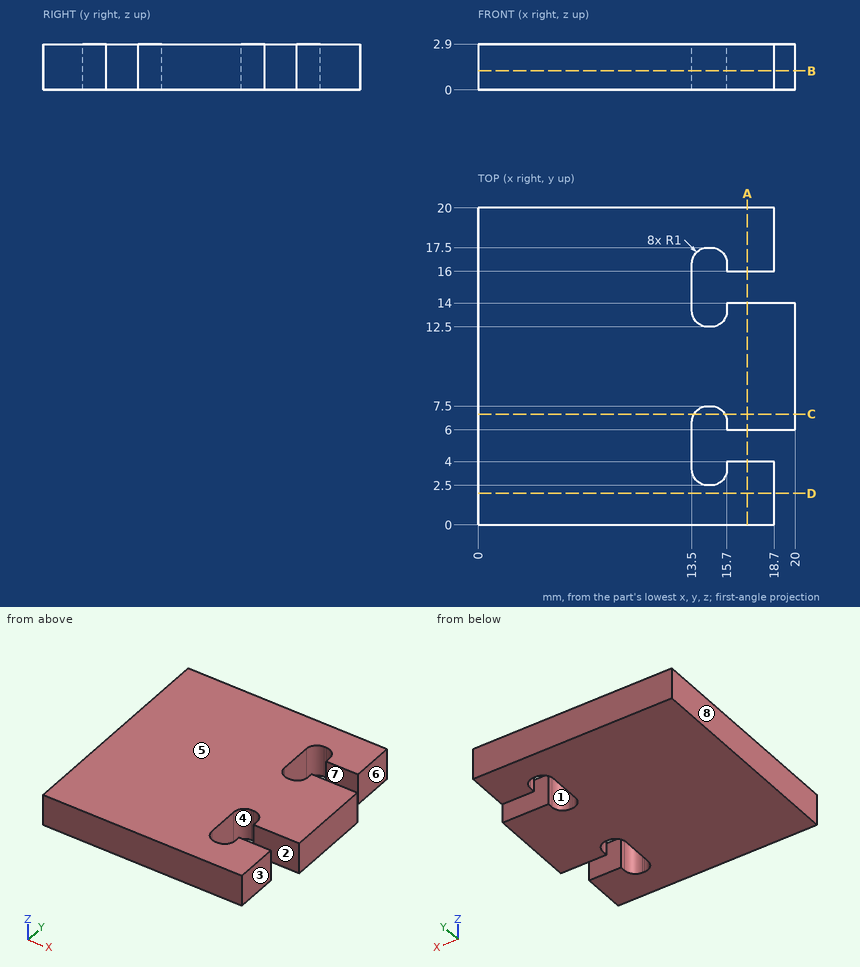
Source: three-view drawing plus pictorial views. Frame: mm from the lowest corner of the part. A direction names the side the tool comes from. Coordinates: 2 decimals unless noted, no trailing zeros. Order: outer loops, then holes, each group sorted by start corner. A loop starts at its lowest first (then second) coordinate and runs counter-clockwise, first axis right, second up.
Item 1: Cut plane B-B (z = 1.2). Return loops of the section in (x, y).
Output values:
outline: (0, 0) - (18.7, 0) - (18.7, 4) - (15.7, 4) - (15.7, 3.5) arc R1 cw to (14.7, 2.5) - (14.5, 2.5) arc R1 cw to (13.5, 3.5) - (13.5, 6.5) arc R1 cw to (14.5, 7.5) - (14.7, 7.5) arc R1 cw to (15.7, 6.5) - (15.7, 6) - (20, 6) - (20, 14) - (15.7, 14) - (15.7, 13.5) arc R1 cw to (14.7, 12.5) - (14.5, 12.5) arc R1 cw to (13.5, 13.5) - (13.5, 16.5) arc R1 cw to (14.5, 17.5) - (14.7, 17.5) arc R1 cw to (15.7, 16.5) - (15.7, 16) - (18.7, 16) - (18.7, 20) - (0, 20) - close
Item 2: Pull-direction query (X, two-part tool) for the marked faces 1, 2 and 3; classes: pulls with the +X half, pulls with the -X half, needs draft (parallel to the pull), parting line crosses it, or undercut.
Output values:
face 1: undercut
face 2: needs draft
face 3: pulls with the +X half
Item 3: Cut plane A-A (x = 17). Return loops of the section in (y, z), plus the area to 3 significant figures.
Output values:
outline: (0, 0) - (4, 0) - (4, 2.9) - (0, 2.9) - close; (6, 0) - (14, 0) - (14, 2.9) - (6, 2.9) - close; (16, 0) - (20, 0) - (20, 2.9) - (16, 2.9) - close
area: 46.4 mm2
Item 4: Material intervals for line 1 (Y direction, x = 16.5, z = 2.5); line 2 (X direction, y = 3.5, z = 1); line 3 (X direction, y = 5.5, z = 0.65), sorted ascending.
Output values:
line 1: y = 0 to 4, 6 to 14, 16 to 20
line 2: x = 0 to 13.5, 15.7 to 18.7
line 3: x = 0 to 13.5
Item 5: Cut plane D-D (y = 2). Return loops of the section in (x, z), plus the area to 3 significant figures.
Output values:
outline: (0, 0) - (18.7, 0) - (18.7, 2.9) - (0, 2.9) - close
area: 54.2 mm2
Item 6: Cut plane C-C (y = 7). Return loops of the section in (x, z), plus the area to 3 significant figures.
Output values:
outline: (0, 0) - (13.63, 0) - (13.63, 2.9) - (0, 2.9) - close; (15.57, 0) - (20, 0) - (20, 2.9) - (15.57, 2.9) - close
area: 52.4 mm2
Item 7: Set-up query: the marked faces 4, 5, 6, 7 and 8. Return all of +Z, -Z, +X, -X, +Y, -Y with unobstructed straight access to the full face (end or side cutting, diameter ignored); none if empty.
Output values:
face 4: +Z, -Z
face 5: +Z, +X, -X, +Y, -Y
face 6: +Z, -Z, +X, +Y
face 7: +Z, -Z, +X
face 8: +Z, -Z, -X, +Y, -Y
